Could you check a few things on this model? Use its own coordinates, in mm. Face numbers are marked on the shaded views. A direction names the side the tool comes from. Round coordinates to 2 decimals unless told otherwise and drop trailing zeros. Loops run counter-clockwise (first coordinate to the right, second up) from the corner with the lowest first, then second, coordinate; pieces in that order, holes last.
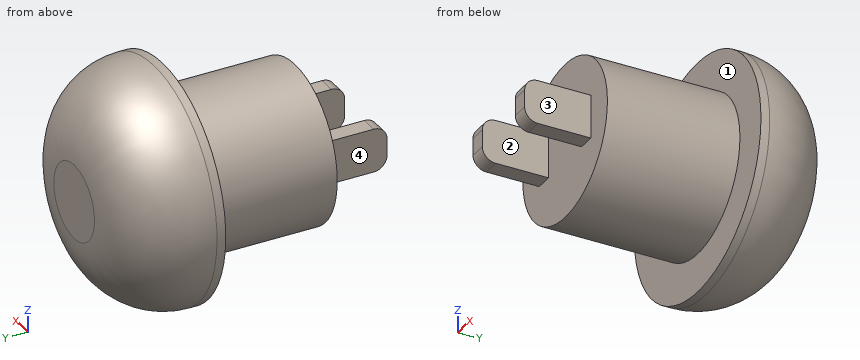
from build123d import *

# Parameters (mm, degrees)
SKETCH1_R           = 5.9
BOSS_EXTRUDE1_DEPTH = 10
SKETCH2_R           = 8.83
BOSS_EXTRUDE2_DEPTH = 6.66
FILLET1_R           = 6
SKETCH3_W           = 1.3
SKETCH3_H           = 1.65
BOSS_EXTRUDE3_DEPTH = 5
FILLET2_R           = 1


with BuildPart() as part:
    # Sketch1 → Boss-Extrude1 (new body)
    with BuildSketch(Plane(origin=(0, 0, 0), x_dir=(1, 0, 0), z_dir=(0, 1, 0))):
        with Locations(Location((0, 0, 0), (0, 0, 270))):
            Circle(SKETCH1_R)
    extrude(amount=BOSS_EXTRUDE1_DEPTH)

    # Sketch2 → Boss-Extrude2 (add)
    with BuildSketch(Plane(origin=(0, 10, 0), x_dir=(1, 0, 0), z_dir=(0, 1, 0))):
        with Locations(Location((0, 0, 0), (0, 0, 270))):
            Circle(SKETCH2_R)
    extrude(amount=BOSS_EXTRUDE2_DEPTH)

    # Fillet1
    fillet1_edges = [part.edges().sort_by_distance(p)[0] for p in [
        (0, 16.66, -8.83),
    ]]
    fillet(fillet1_edges, radius=FILLET1_R)

    # Sketch3 → Boss-Extrude3 (add)
    with BuildSketch(Plane.XZ):
        with Locations((2.95, -0.825)):
            Rectangle(SKETCH3_W, SKETCH3_H)
        with Locations((2.95, 0.825)):
            Rectangle(SKETCH3_W, SKETCH3_H)
        with Locations((-2.95, 0.825)):
            Rectangle(SKETCH3_W, SKETCH3_H)
        with Locations((-2.95, -0.825)):
            Rectangle(SKETCH3_W, SKETCH3_H)
    extrude(amount=BOSS_EXTRUDE3_DEPTH)

    # Fillet2
    fillet2_edges = [part.edges().sort_by_distance(p)[0] for p in [
        (2.95, -5, -1.65),
        (2.95, -5, 1.65),
        (-2.95, -5, 1.65),
        (-2.95, -5, -1.65),
    ]]
    fillet(fillet2_edges, radius=FILLET2_R)


solid = part.part
Item 1: For the marked faces 1, 2, 3 and 4, which set-ups out of +Z, -Z, +X, -X, +Y, -Y let a thin tool reach every point of the face, with its end or its side?
Results list:
face 1: -Y
face 2: +Z, -Z, -Y
face 3: +Z, -Z, +X, -Y
face 4: +Z, -Z, -X, -Y
Item 2: If we section it at A-A, the plane y = 4.75: Please give me the cut outline in (x, z).
Results list:
outline: circle Ø11.8 at (0, 0)
Item 3: Will these pins go through, and if not, where does the flat tip stop? pin 1 (5 mm diameter, centred on y = 3.5, z = 4.5, fed in from +X); pin 2 (1 mm diameter, centred on x = -2.5, y = -1, fed in from +Z); pin 3 (1 mm diameter, centred on x = -3, y = -2, fed in from -Z).
Results list:
pin 1: stops at x = 5.55
pin 2: stops at z = 1.65
pin 3: stops at z = -1.65
Item 4: If I drill on line 1 along X through (y, z) = (-2.75, 1); line 2 along Y through (x, z) = (-1.75, 1.5); line 3 along Z through (x, y) = (1, 9.5), over which ranges is the centre line in solid material (lowest first)?
Results list:
line 1: x = -3.6 to -2.3, 2.3 to 3.6
line 2: y = 0 to 16.66
line 3: z = -5.81 to 5.81
